Read the model definition and answer for the solid it produces. Units are mm, in the model's axes. Give positions to 0.01 mm unless a question says otherwise; leave off trailing zeros. Loops run counter-clockwise (first coordinate to the right, second up) from the corner with the lowest first, then second, coordinate; pieces in that order, holes last.
(1) Find section B-B, the plane x = 0. Write down the section's boundary in (y, z).
(2) Find section C-C, the plane z = -8.5. Write down the section's boundary in (x, y), then the cut area to 3 significant figures.
(3) Find section D-D, the plane x = 4.82. Write down the section's boundary in (y, z).
(4) Each of these flat-tipped pins is pushed along its axis until it touches: P1, Ø0.5, axis at x = 0, y = 0, coming from the -Z side; P2, Ø2, axis at x = 0.5, z = -5.5, coming from the -Y side. Where does it stop, or does it pass through?
(5) Find section A-A, the plane y = 46.6. Write down the section's boundary in (x, z), then the cut area to 3 significant figures.
(6) A straight line is drawn through the part: probe 1 along Y at (x, z) = (0, -10.5). Find the intervals that lie inside material, in ascending order.
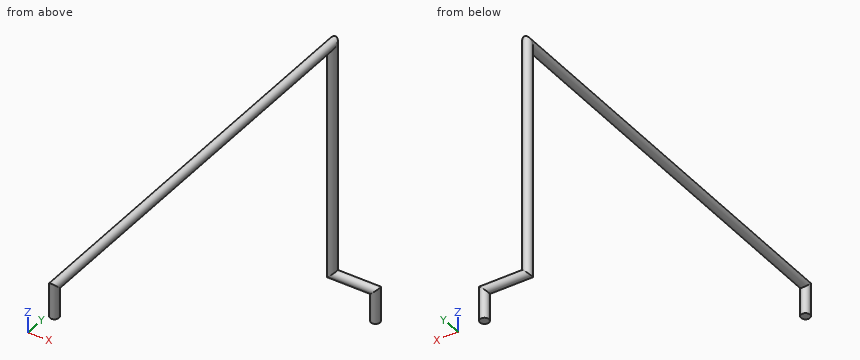
```python
from build123d import *

# Parameters (mm, degrees)
ESQUISSE2_R = 0.5


with BuildPart() as part:
    # Balayage2: sweep along a curve in space
    with BuildLine() as balayage2_path:
        Line((0, 0, 0), (0, 0, 3.5))
        Line((0, 0, 3.5), (0, 46.6, 3.5))
        Line((0, 46.6, 3.5), (0, 46.6, -22.89))
        Line((0, 46.6, -22.89), (4.82, 46.6, -22.89))
        Line((4.82, 46.6, -22.89), (4.82, 46.6, -26.39))
    # Esquisse2 → Balayage2 (sweep)
    with BuildSketch(Plane.XY):
        Circle(ESQUISSE2_R)
    sweep(path=balayage2_path.line, transition=Transition.RIGHT)


solid = part.part
```
Entries:
1. outline: (-0.5, 0) - (0.5, 0) - (0.5, 3) - (46.1, 3) - (46.1, -22.89) arc R0.5 ccw to (47.1, -22.89) - (47.1, 4) - (-0.5, 4) - close
2. outline: circle Ø1 at (0, 46.6)
2. area: 0.785 mm2
3. outline: (46.1, -26.39) - (47.1, -26.39) - (47.1, -22.89) arc R0.5 ccw to (46.1, -22.89) - close
4. P1: stops at z = 0
4. P2: stops at y = 46.1
5. outline: (-0.5, -23.39) - (4.32, -23.39) - (4.32, -26.39) - (5.32, -26.39) - (5.32, -22.39) - (0.5, -22.39) - (0.5, 3.5) arc R0.5 ccw to (-0.5, 3.5) - close
5. area: 35.1 mm2
6. probe 1: y = 46.1 to 47.1
